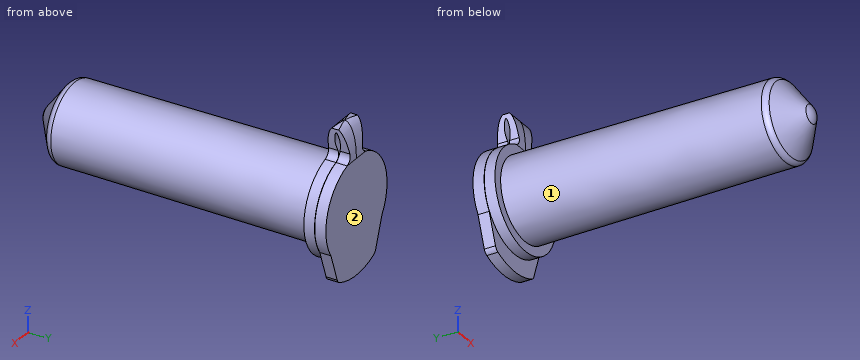
```python
from build123d import *

# Parameters (mm, degrees)
BOSS_EXTRUDE1_DEPTH     = 1.47
BOSS_EXTRUDE2_REACH     = 44.45
CUT_EXTRUDE1_DEPTH      = 40.240986748
CUT_EXTRUDE1_DEPTH_BACK = 40.240986748


with BuildPart() as part:
    # Sketch1 → Revolve1 (revolve)
    with BuildSketch(Plane.XY, mode=Mode.PRIVATE) as revolve1_sk:
        with BuildLine():
            Line((1.192198173, -3.462113799), (4.773990196, -0.802910879))
            ThreePointArc((4.773990196, -0.802910879), (5.069930367, -0.451957922), (5.177874547, -0.005755483))
            Line((5.177874547, -0.005755483), (5.375, 34.243707959))
            Line((5.375, 34.243707959), (6.6, 34.243707959))
            Line((6.6, 34.243707959), (6.6, 35.643707959))
            Line((6.6, 35.643707959), (5.128724562, 35.643707959))
            Line((5.128724562, 35.643707959), (4.378724562, 34.893707959))
            Line((4.378724562, 34.893707959), (4.17789111, 0))
            Line((4.17789111, 0), (0.596099086, -2.65920292))
            ThreePointArc((0.596099086, -2.65920292), (0.31391808, -2.805742113), (0, -2.856292041))
            Line((0, -2.856292041), (0, -3.856292041))
            ThreePointArc((0, -3.856292041), (0.627836159, -3.755192185), (1.192198173, -3.462113799))
        make_face()
        Polygon((4.25, 32.893707959), (4.25, 36.393707959), (6, 36.393707959), (6, 35.673707959), (6.6, 35.673707959), (6.6, 36.140431751), (6.6, 37.143707959), (0, 37.143707959), (0, 36.393707959), (3.65, 36.393707959), (3.65, 32.893707959), align=None)
    revolve(revolve1_sk.sketch.rotate(Axis((0, 0, 0), (0, 1, 0)), 90), axis=Axis((0, 0, 0), (0, 1, 0)))

    # Sketch2 → Boss-Extrude1 (add)
    with BuildSketch(Plane(origin=(0, 37.143707959, 0), x_dir=(1, 0, 0), z_dir=(0, 1, 0))):
        with BuildLine():
            Line((-5.5, 3.648287269), (-4.147964107, 7.446102732))
            ThreePointArc((-4.147964107, 7.446102732), (-3.941225776, 7.788413444), (-3.616893324, 8.02234895))
            ThreePointArc((-3.616893324, 8.02234895), (0, 8.8), (3.616893324, 8.02234895))
            ThreePointArc((3.616893324, 8.02234895), (3.941225776, 7.788413444), (4.147964107, 7.446102732))
            Line((4.147964107, 7.446102732), (5.5, 3.648287269))
            ThreePointArc((5.5, 3.648287269), (0, 6.6), (-5.5, 3.648287269))
        make_face()
    extrude(amount=-BOSS_EXTRUDE1_DEPTH)

    # Boss-Extrude2: up to this face of the body (flat: up to its plane)
    boss_extrude2_end = Plane(part.part.faces().sort_by_distance((0, 34.243707959, 5.56167619))[0])
    # Sketch3 → Boss-Extrude2 (add, up to the picked face)
    with BuildSketch(Plane(origin=(0, 37.143707959, 0), x_dir=(1, 0, 0), z_dir=(0, 1, 0)), mode=Mode.PRIVATE) as boss_extrude2_sk1:
        with BuildLine():
            Line((0, -6.6), (0, -10.8))
            ThreePointArc((0, -10.8), (1.019553267, -10.751767814), (2.03, -10.607502062))
            ThreePointArc((2.03, -10.607502062), (1.706052324, -9.043133027), (1.335, -7.489262778))
            ThreePointArc((1.335, -7.489262778), (1.429653992, -6.757094078), (2.000871697, -6.289396828))
            ThreePointArc((2.000871697, -6.289396828), (1.01241813, -6.521886961), (0, -6.6))
        make_face()
    boss_extrude2_tool1 = split(extrude(boss_extrude2_sk1.sketch, amount=-BOSS_EXTRUDE2_REACH, mode=Mode.PRIVATE), bisect_by=boss_extrude2_end, keep=Keep.BOTH, mode=Mode.PRIVATE)
    # Sketch3 → Boss-Extrude2 (add, up to the picked face)
    with BuildSketch(Plane(origin=(0, 37.143707959, 0), x_dir=(1, 0, 0), z_dir=(0, 1, 0)), mode=Mode.PRIVATE) as boss_extrude2_sk2:
        with BuildLine():
            ThreePointArc((-2.03, -10.607502062), (-1.019553267, -10.751767814), (0, -10.8))
            Line((0, -10.8), (0, -6.6))
            ThreePointArc((0, -6.6), (-1.01241813, -6.521886961), (-2.000871697, -6.289396828))
            ThreePointArc((-2.000871697, -6.289396828), (-1.429653992, -6.757094078), (-1.335, -7.489262778))
            ThreePointArc((-1.335, -7.489262778), (-1.706052324, -9.043133027), (-2.03, -10.607502062))
        make_face()
    boss_extrude2_tool2 = split(extrude(boss_extrude2_sk2.sketch, amount=-BOSS_EXTRUDE2_REACH, mode=Mode.PRIVATE), bisect_by=boss_extrude2_end, keep=Keep.BOTH, mode=Mode.PRIVATE)
    add(boss_extrude2_tool1.solids().sort_by(Axis((0.832919, 37.143708, 8.79495), (0, -1, 0)))[0])
    add(boss_extrude2_tool2.solids().sort_by(Axis((-0.832919, 37.143708, 8.79495), (0, -1, 0)))[0])

    # Sketch5 → Cut-Extrude1 (cut, two sides)
    with BuildSketch(Plane(origin=(0, 0, 0), x_dir=(0, 0, -1), z_dir=(1, 0, 0))) as cut_extrude1_sk:
        with BuildLine():
            Line((-6.289396828, 35.643707959), (-6.6, 35.643707959))
            add(Edge.make_bspline(
                [(-6.6, 35.673707959), (-7.519037203, 35.673707959), (-8.421750075, 36.327077496), (-10.369945566, 35.658707959), (-8.421586809, 34.990338421), (-7.521291173, 35.643707959), (-6.6, 35.643707959)],
                knots=[0, 0, 0, 0, 0.417765924, 0.5, 0.582234076, 1, 1, 1, 1], degree=3))
            Line((-6.6, 35.673707959), (-6.289396828, 35.673707959))
            Line((-6.289396828, 35.673707959), (-6.289396828, 35.643707959))
        make_face()
        with BuildLine():
            Line((-6.289396828, 34.243707959), (-6.289396828, 33.533396672))
            Line((-6.289396828, 33.533396672), (-11.467394827, 33.825492735))
            Line((-11.467394827, 33.825492735), (-11.357937817, 38.544473635))
            Line((-11.357937817, 38.544473635), (-6.289396828, 38.035452095))
            Line((-6.289396828, 38.035452095), (-6.289396828, 37.143707959))
            add(Edge.make_bspline(
                [(-6.289396828, 37.143707959), (-9.431918588, 37.143707959), (-12.135369897, 35.479054802), (-9.496663947, 34.243707959), (-6.289396828, 34.243707959)],
                knots=[0, 0, 0, 0, 0.503821902, 1, 1, 1, 1], degree=3))
        make_face()
    extrude(amount=CUT_EXTRUDE1_DEPTH, mode=Mode.SUBTRACT)
    extrude(cut_extrude1_sk.sketch, amount=-CUT_EXTRUDE1_DEPTH_BACK, mode=Mode.SUBTRACT)


solid = part.part
```
Source: CAD feature listing. Evaluate the final solid. Frame: model axes, mm. Face numbers are marked on the shaded views. A direction names the side the tool comes from. Give positions to 0.01 mm unless a question says otherwise; leave off trailing zeros. Write each loop counter-clockwise with the first axis right and the second up, starting at its lowest first coordinate (ties: lowest second). Pieces come first, ordered by that corner, then holes.
1. Section query A-A (y = 10). Return the cut outline in (x, z), then the cut area to 3 significant figures.
2. First-contact query: pin 1 (10 mm diameter, centred on y = 4, z = -3.5, fed in from -X); pin 2 (2 mm diameter, centred on x = -1.5, z = -0.5, fed in from -Y); pin 3 (6 mm diameter, centred on x = 0, z = 3, fed in from -Y); pin 4 (1 mm diameter, centred on x = 0.5, z = 9, fed in from +Y). Flat tips, straight axial feed; report the tip coordinate or a pass-through.
3. Material intervals for line 1 along X through (y, z) = (36, 0); line 2 along Y through (x, z) = (1, -5.75); line 3 along Z through (x, y) = (-0.75, 10.5), sorted ascending.
4. Section query B-B (y = 3). Return the cut outline in (x, z).
5. Access query for the marked faces 1 and 2. Directions: +Z, -Z, +X, -X, +Y, -Y. A direction counts if a zero-diameter tool reaches every point of the face in a straight line with its end or side. Return the directions, or none.
Output values:
1. outline: circle Ø10.47 at (0, 0); hole circle Ø8.47 at (0, 0)
1. area: 29.8 mm2
2. pin 1: stops at x = -5.22
2. pin 2: stops at y = -3.77
2. pin 3: stops at y = -3.86
2. pin 4: stops at y = 36.97
3. line 1: x = -6.6 to -6, -4.25 to -3.65, 3.65 to 4.25, 6 to 6.6
3. line 2: y = 34.24 to 35.64, 36.39 to 37.14
3. line 3: z = -5.18 to -4.17, 4.17 to 5.18
4. outline: circle Ø10.39 at (0, 0); hole circle Ø8.39 at (0, 0)
5. face 1: -Y
5. face 2: +Z, -Z, +X, -X, +Y
